Design review of the part built by this model. Coordinates are the model's own, in mm. A direction names the side the tool comes from. Coordinates: 2 decimals unless noted, no trailing zeros. Loops run counter-clockwise (first coordinate to the right, second up) from the corner with the lowest first, then second, coordinate; pieces in that order, holes last. Notation, with made-up numbers: (8, -24) - (19, -24) arc R26 cw to (19, 10) - close; hole circle Ø3 at (51.5, 39). An arc over 180 degrees is marked (long way). Return JSON: item names as keys, results as strings. Group by question number.
from build123d import *

# Parameters (mm, degrees)
BOSS_EXTRUDE1_DEPTH  = 5
SKETCH2_W            = 2
SKETCH2_H            = 10
CUT_EXTRUDE1_DEPTH   = 151
SKETCH3_R            = 1.75
SKETCH3_R_2          = 1.5
SKETCH3_R_3          = 1.65
SKETCH3_R_4          = 0.785
CUT_EXTRUDE2_DEPTH   = 6
SKETCH4_R            = 2
CUT_EXTRUDE3_DEPTH   = 2.5
SKETCH5_R            = 1.25
CUT_EXTRUDE4_DEPTH   = 3.5
LPATTERN1_COUNT      = 3
LPATTERN1_PITCH      = 10
LPATTERN1_COUNT_DIR2 = 2
LPATTERN1_PITCH_DIR2 = 80


with BuildPart() as part:
    # Sketch1 → Boss-Extrude1 (new body)
    with BuildSketch(Plane.XY):
        Polygon((72, -17.5), (75, -14.5), (75, 17.5), (-75, 17.5), (-75, -14.5), (-72, -17.5), align=None)
    extrude(amount=BOSS_EXTRUDE1_DEPTH)

    # Sketch2 → Cut-Extrude1 (cut, through all)
    with BuildSketch(Plane(origin=(75, 0, 0), x_dir=(0, 0, -1), z_dir=(1, 0, 0))):
        with Locations((-4, 12.5)):
            Rectangle(SKETCH2_W, SKETCH2_H)
    extrude(amount=-CUT_EXTRUDE1_DEPTH, mode=Mode.SUBTRACT)

    # Sketch3 → Cut-Extrude2 (cut, through all)
    with BuildSketch(Plane(origin=(0, 0, 0), x_dir=(-1, 0, 0), z_dir=(0, 0, -1))):
        with Locations((-65, 12.5)):
            Circle(SKETCH3_R)
        with Locations((65, 12.5)):
            Circle(SKETCH3_R)
        with Locations((-44.5, 2.5)):
            Circle(SKETCH3_R_2)
        with Locations((-39.5, 2.5)):
            Circle(SKETCH3_R_3)
        with Locations((-46.5, -15)):
            Circle(SKETCH3_R_4)
        with Locations((-38.5, -15)):
            Circle(SKETCH3_R_4)
        with Locations((-32, -5.5)):
            Circle(SKETCH3_R)
        with Locations((-32, -13.5)):
            Circle(SKETCH3_R)
        with Locations((48, -5.5)):
            Circle(SKETCH3_R)
        with Locations((48, -13.5)):
            Circle(SKETCH3_R)
        with Locations((67.5, 2.5)):
            Circle(SKETCH3_R_2)
        with Locations((72.5, 2.5)):
            Circle(SKETCH3_R_3)
    extrude(amount=-CUT_EXTRUDE2_DEPTH, mode=Mode.SUBTRACT)

    # Sketch4 → Cut-Extrude3 (cut)
    with BuildSketch(Plane(origin=(0, 0, 0), x_dir=(-1, 0, 0), z_dir=(0, 0, -1))):
        with Locations((-24, 5)):
            Circle(SKETCH4_R)
    cut_extrude3 = extrude(amount=-CUT_EXTRUDE3_DEPTH, mode=Mode.SUBTRACT)

    # Sketch5 → Cut-Extrude4 (cut, through all)
    with BuildSketch(Plane(origin=(0, 0, 2.5), x_dir=(-1, 0, 0), z_dir=(0, 0, -1))):
        with Locations((-24, 5)):
            Circle(SKETCH5_R)
    cut_extrude4 = extrude(amount=-CUT_EXTRUDE4_DEPTH, mode=Mode.SUBTRACT)

    # LPattern1: Cut-Extrude3, Cut-Extrude4 3 × 2
    with Locations(*[(-j * LPATTERN1_PITCH_DIR2, -i * LPATTERN1_PITCH, 0) for i in range(LPATTERN1_COUNT) for j in range(LPATTERN1_COUNT_DIR2) if (i, j) != (0, 0)]):
        add(cut_extrude3, mode=Mode.SUBTRACT)
        add(cut_extrude4, mode=Mode.SUBTRACT)


solid = part.part
Item 1: Add section A-A (x = 32). State the section outline as (y, z) points.
Item 2: Add section B-B (x = -42.5). State the section outline as (y, z) points, then the cut area to 3 significant figures.
Item 3: Draft analysis for pull direction Y (two halves, no side actions). For faces 3 (the face through (-73.5, -16, 2.5)), 4 (the face through (-49.617, -6.17, 2.465)), 5 (the face through (-1, 0, 0)), 6 (the face through (-68.93, 2.95, 2.46)), state which applies: pulls with the +Y half, pulls with the -Y half, needs draft (parallel to the pull), parting line crosses it, or undercut.
Item 4: For P1, Ø5, axis at x = 46, y = 5.5, coming from the -Z side; P2, Ø0.6, axis at x = 13.5, z = 4.5, coming from the +Y side; P3, Ø2, axis at x = -55.5, y = 5.5, coming from the -Z side; P4, Ø3, axis at x = -48, y = -13.5, coming from the +Z side, all flat-tipped, find the tip position at first contact; note any pin that passes through.
Item 5: For faces 1 (the face through (-1, -17.5, 2)), 2 (the face through (-55, -16, 2.5)), list the 3-axis set-ups (+Z, -Z, +X, -X, +Y, -Y) from which the entire face can be reached by the end or side of a thin tool; tool diameter is ignored.
Item 6: To check wall thickness, follow line 1 (Y direction, x = 24, z = 1.95); line 2 (Y direction, x = -56, z = 4.25); line 3 (Y direction, x = 32, z = 1.1). State the ranges of each line that lie inside material, in increasing order. Write a range as from..to.
Answers below:
{
 "1": {"outline": "(-17.5, 0) - (-15.25, 0) - (-15.25, 5) - (-17.5, 5) - close; (-11.75, 0) - (-7.25, 0) - (-7.25, 5) - (-11.75, 5) - close; (-3.75, 0) - (17.5, 0) - (17.5, 3) - (7.5, 3) - (7.5, 5) - (-3.75, 5) - close"},
 "2": {"outline": "(-17.5, 0) - (17.5, 0) - (17.5, 3) - (7.5, 3) - (7.5, 5) - (-17.5, 5) - close", "area": "155 mm^2"},
 "3": {"face 3": "pulls with the -Y half", "face 4": "undercut", "face 5": "needs draft", "face 6": "undercut"},
 "4": {"P1": "stops at z = 0", "P2": "stops at y = 7.5", "P3": "stops at z = 2.5", "P4": "passes through"},
 "5": {"face 1": "+Z, -Z, +X, -X, -Y", "face 2": "-Z"},
 "6": {"line 1": "y = -17.5..-17, -13..-7, -3..3, 7..17.5", "line 2": "y = -17.5..-16.25, -13.75..-6.25, -3.75..3.75, 6.25..7.5", "line 3": "y = -17.5..-15.25, -11.75..-7.25, -3.75..17.5"}
}
